Verification items for the finished model (mm, model axes). A direction names the side the tool comes from. Round coordinates to 2 decimals unless told otherwise and drop trailing zeros. Order: outer loops, then holes, each group sorted by start corner. A loop starts at its lowest first (then second) coordinate and runs counter-clockwise, first axis right, second up. Notation, with made-up numbers: M 25.25,16 L 60.25,16 A5 cw 60.25,21 Z; hole C 55,-23 d2. An arc over 180 degrees is marked long. Answer as a JSON object with one key per item and string values. Group by question number.
```python
from build123d import *
from build123d.topology import SkipClean

# Parameters (mm, degrees)
SKETCH_1_R                       = 40
EXTRUDE_1_DEPTH                  = 150
SKETCH_2_R                       = 55
EXTRUDE_2_DEPTH                  = 50
SKETCH_3_R                       = 30
CUT_EXTRUDE_2_DEPTH              = 200
CUT_EXTRUDE_3_DEPTH              = 134
CUT_EXTRUDE_3_DEPTH_BACK         = 106
SKETCH_5_R                       = 6
EXTRUDE_3_DEPTH                  = 45
SKETCH_15_R                      = 50
EXTRUDE_5_DEPTH                  = 20
EXTRUDE_6_DEPTH                  = 59.991870163
SKETCH_17_R                      = 40
EXTRUDE_7_DEPTH                  = 30
SKETCH_18_R                      = 26
CUT_EXTRUDE_25_DEPTH             = 30
SKETCH_19_R                      = 17
CUT_EXTRUDE_26_DEPTH             = 51
CUT_EXTRUDE_27_DEPTH             = 170
CUT_EXTRUDE_27_DEPTH_BACK        = 99
SKETCH_20_R                      = 30
SKETCH_21_R                      = 25
CUT_EXTRUDE_28_DEPTH             = 60
EXTRUDE_8_DEPTH                  = 28
EXTRUDE_8_DEPTH_BACK             = 28
SKETCH_23_R                      = 8.294671539
CUT_EXTRUDE_29_DEPTH             = 70
CUT_EXTRUDE_30_REACH             = 185.367
CUT_EXTRUDE_30_END_RADIUS        = 55
SKETCH_24_W                      = 85
SKETCH_24_H                      = 25
CUT_EXTRUDE_30_DIRECTION_2_DEPTH = 70
CUT_EXTRUDE_31_DEPTH             = 70
CUT_EXTRUDE_31_DEPTH_BACK        = 70
SKETCH_25_W                      = 85
SKETCH_25_H                      = 25
SKETCH_26_R                      = 26
CUT_EXTRUDE_32_DEPTH             = 30
SKETCH_27_R                      = 17
CUT_EXTRUDE_33_DEPTH             = 55
CUT_EXTRUDE_34_DEPTH             = 417
CUT_EXTRUDE_34_DEPTH_BACK        = 195
SKETCH_29_R                      = 30


with BuildPart() as part:
    # 草图1 → 凸台-拉伸1 (new body)
    with BuildSketch(Plane(origin=(0, 0, 0), x_dir=(0, 0, -1), z_dir=(1, 0, 0))):
        Circle(SKETCH_1_R)
    extrude(amount=EXTRUDE_1_DEPTH)

    # 草图2 → 凸台-拉伸2 (add)
    with BuildSketch(Plane(origin=(0, 0, 0), x_dir=(0, 0, -1), z_dir=(1, 0, 0))):
        Circle(SKETCH_2_R)
    extrude(amount=-EXTRUDE_2_DEPTH)

    # 草图3 → 切除-拉伸2 (cut)
    with BuildSketch(Plane(origin=(150, 0, 0), x_dir=(0, 0, -1), z_dir=(1, 0, 0))):
        Circle(SKETCH_3_R)
    extrude(amount=-CUT_EXTRUDE_2_DEPTH, mode=Mode.SUBTRACT)

    # 草图5 → 切除-拉伸3 (cut, two sides: drawn at the far end of the back side and taken through both)
    with BuildSketch(Plane.XY.offset(-CUT_EXTRUDE_3_DEPTH_BACK)):
        with Locations((-25, 0)):
            Circle(SKETCH_5_R)
    extrude(amount=CUT_EXTRUDE_3_DEPTH + CUT_EXTRUDE_3_DEPTH_BACK, mode=Mode.SUBTRACT)

    # 草图7 → 凸台-拉伸3 (add)
    with BuildSketch(Plane(origin=(0, 0, 0), x_dir=(1, 0, 0), z_dir=(0, 1, 0))):
        with BuildLine():
            Line((82.442023832, 21.548591956), (100.118268858, 21.548591956))
            ThreePointArc((100.118268858, 21.548591956), (105, 0), (100.118268858, -21.548591956))
            Line((100.118268858, -21.548591956), (82.442023832, -21.548591956))
            ThreePointArc((82.442023832, -21.548591956), (55, -34.891352615), (27.557976168, -21.548591956))
            Line((27.557976168, -21.548591956), (9.881731142, -21.548591956))
            ThreePointArc((9.881731142, -21.548591956), (5, 0), (9.881731142, 21.548591956))
            Line((9.881731142, 21.548591956), (27.557976168, 21.548591956))
            ThreePointArc((27.557976168, 21.548591956), (55, 34.891352615), (82.442023832, 21.548591956))
        make_face()
    extrude(amount=EXTRUDE_3_DEPTH)

    # 草图15 → 凸台-拉伸5 (add)
    with SkipClean():  # the faces are left unmerged after this step: merging them gives an invalid solid
        with BuildSketch(Plane(origin=(0, 45, 0), x_dir=(1, 0, 0), z_dir=(0, 1, 0))):
            with Locations(Location((55, 0, 0), (0, 0, 154.470748686))):
                Circle(SKETCH_15_R)
        extrude(amount=EXTRUDE_5_DEPTH)

    # 草图16 → 凸台-拉伸6 (add)
    with SkipClean():  # the faces are left unmerged after this step: merging them gives an invalid solid
        with BuildSketch(Plane(origin=(0, 0, 0), x_dir=(1, 0, 0), z_dir=(0, 1, 0))):
            with BuildLine():
                Line((30.539216555, 13.626080627), (17.392421951, 13.626080627))
                ThreePointArc((17.392421951, 13.626080627), (15, 0), (17.392421951, -13.626080627))
                Line((17.392421951, -13.626080627), (30.539216555, -13.626080627))
                ThreePointArc((30.539216555, -13.626080627), (55, -28), (79.460783445, -13.626080627))
                Line((79.460783445, -13.626080627), (92.607578049, -13.626080627))
                ThreePointArc((92.607578049, -13.626080627), (95, 0), (92.607578049, 13.626080627))
                Line((92.607578049, 13.626080627), (79.460783445, 13.626080627))
                ThreePointArc((79.460783445, 13.626080627), (55, 28), (30.539216555, 13.626080627))
            make_face()
        extrude(amount=-EXTRUDE_6_DEPTH)

    # 草图17 → 凸台-拉伸7 (add)
    with BuildSketch(Plane.XZ.offset(59.991870163)):
        with Locations(Location((55, 0, 0), (0, 0, 19.916603358))):
            Circle(SKETCH_17_R)
    extrude(amount=EXTRUDE_7_DEPTH)

    # 草图18 → 切除-拉伸25 (cut)
    with BuildSketch(Plane.XZ.offset(89.991870163)):
        with Locations(Location((55, 0, 0), (0, 0, 270))):
            Circle(SKETCH_18_R)
    extrude(amount=-CUT_EXTRUDE_25_DEPTH, mode=Mode.SUBTRACT)

    # 草图19 → 切除-拉伸26 (cut)
    with BuildSketch(Plane.XZ.offset(59.991870163)):
        with Locations(Location((55, 0, 0), (0, 0, 270))):
            Circle(SKETCH_19_R)
    extrude(amount=-CUT_EXTRUDE_26_DEPTH, mode=Mode.SUBTRACT)

    # 草图20 → 切除-拉伸27 (cut, two sides: drawn at the far end of the back side and taken through both)
    with BuildSketch(Plane(origin=(0, 0, 0), x_dir=(0, 0, -1), z_dir=(1, 0, 0)).offset(-CUT_EXTRUDE_27_DEPTH_BACK)):
        Circle(SKETCH_20_R)
    extrude(amount=CUT_EXTRUDE_27_DEPTH + CUT_EXTRUDE_27_DEPTH_BACK, mode=Mode.SUBTRACT)

    # 草图21 → 切除-拉伸28 (cut)
    with BuildSketch(Plane(origin=(0, 65, 0), x_dir=(1, 0, 0), z_dir=(0, 1, 0))):
        with Locations(Location((55, 0, 0), (0, 0, 270))):
            Circle(SKETCH_21_R)
    extrude(amount=-CUT_EXTRUDE_28_DEPTH, mode=Mode.SUBTRACT)

    # 草图22 → 凸台-拉伸8 (add, two sides: drawn at the far end of the back side and taken through both)
    with BuildSketch(Plane.XY.offset(-EXTRUDE_8_DEPTH_BACK)):
        with BuildLine():
            Line((119.756495452, -72.615787856), (55, -72.615787856))
            Line((55, -72.615787856), (55, -17.615787856))
            Line((55, -17.615787856), (134.756495452, -17.615787856))
            Line((134.756495452, -17.615787856), (134.756495452, -57.615787856))
            ThreePointArc((134.756495452, -57.615787856), (130.36309717, -68.222389574), (119.756495452, -72.615787856))
        make_face()
    extrude(amount=EXTRUDE_8_DEPTH + EXTRUDE_8_DEPTH_BACK)

    # 草图23 → 切除-拉伸29 (cut)
    with BuildSketch(Plane.XY.offset(28)):
        with Locations((118.599166742, -58.702167389)):
            Circle(SKETCH_23_R)
    extrude(amount=-CUT_EXTRUDE_29_DEPTH, mode=Mode.SUBTRACT)

    # 切除-拉伸30: up to this cylinder (the profile starts inside it)
    cut_extrude_30_end = Plane(origin=(-27.5, 0, 0), z_dir=(1, 0, 0)) * Cylinder(CUT_EXTRUDE_30_END_RADIUS, 481.734, mode=Mode.PRIVATE)
    # 草图24 → 切除-拉伸30 (cut, up to the surface)
    with BuildSketch(Plane(origin=(0, 0, 0), x_dir=(1, 0, 0), z_dir=(0, 1, 0)), mode=Mode.PRIVATE) as cut_extrude_30_sk1:
        with Locations((-27.5, -47.5)):
            Rectangle(SKETCH_24_W, SKETCH_24_H)
    cut_extrude_30_tool1 = extrude(cut_extrude_30_sk1.sketch, amount=-CUT_EXTRUDE_30_REACH, mode=Mode.PRIVATE) & cut_extrude_30_end
    add(cut_extrude_30_tool1.solids().sort_by_distance((-27.5, 0, 47.5))[0], mode=Mode.SUBTRACT)

    # 草图24 → 切除-拉伸30 direction 2 (cut)
    with BuildSketch(Plane(origin=(0, 0, 0), x_dir=(1, 0, 0), z_dir=(0, 1, 0))):
        with Locations((-27.5, -47.5)):
            Rectangle(SKETCH_24_W, SKETCH_24_H)
    extrude(amount=CUT_EXTRUDE_30_DIRECTION_2_DEPTH, mode=Mode.SUBTRACT)

    # 草图25 → 切除-拉伸31 (cut, two sides: drawn at the far end of the back side and taken through both)
    with BuildSketch(Plane(origin=(0, 0, 0), x_dir=(1, 0, 0), z_dir=(0, 1, 0)).offset(-CUT_EXTRUDE_31_DEPTH_BACK)):
        with Locations((-27.5, 47.5)):
            Rectangle(SKETCH_25_W, SKETCH_25_H)
    extrude(amount=CUT_EXTRUDE_31_DEPTH + CUT_EXTRUDE_31_DEPTH_BACK, mode=Mode.SUBTRACT)

    # 草图26 → 切除-拉伸32 (cut)
    with BuildSketch(Plane.XZ.offset(89.991870163)):
        with Locations(Location((55, 0, 0), (0, 0, 270))):
            Circle(SKETCH_26_R)
    extrude(amount=-CUT_EXTRUDE_32_DEPTH, mode=Mode.SUBTRACT)

    # 草图27 → 切除-拉伸33 (cut)
    with BuildSketch(Plane.XZ.offset(59.991870163)):
        with Locations(Location((55, 0, 0), (0, 0, 270))):
            Circle(SKETCH_27_R)
    extrude(amount=-CUT_EXTRUDE_33_DEPTH, mode=Mode.SUBTRACT)

    # 草图29 → 切除-拉伸34 (cut, two sides: drawn at the far end of the back side and taken through both)
    with BuildSketch(Plane(origin=(0, 0, 0), x_dir=(0, 0, -1), z_dir=(1, 0, 0)).offset(-CUT_EXTRUDE_34_DEPTH_BACK)):
        Circle(SKETCH_29_R)
    extrude(amount=CUT_EXTRUDE_34_DEPTH + CUT_EXTRUDE_34_DEPTH_BACK, mode=Mode.SUBTRACT)


solid = part.part
```
Q1. Thickness scan on line 1 (Z direction, x = 55, y = -53); line 2 (X direction, y = -61, z = -17); line 3 (X direction, y = 48.5, z = -4.5). Record the ranges inside material, lowest first. Write a range as from..to.
Q2. Cross-section at A-A, the plane x = -25. Record the cut outline in (y, z), then the cut area to 3 significant figures.
Q3. Cross-section at D-D, the plane x = -4. Record the cut outline in (y, z).
Q4. Cross-section at C-C, the plane y = 0. Record the cut outline in (x, z).
Q5. Gauge pin test, flat ends, axial feed: pin 1 Ø4 at (x, y) = (98, -34) entering from -Z; pin 2 Ø6 at (x, y) = (-29, -50) entering from -Z; pin 3 Ø12 at (x, y) = (-23, -20) entering from -Z; pin 4 Ø9.5 at (x, y) = (-25, 0) entering from +Z. Record the tip position at first contact, or that the pin passes through.
Q6. Release check for a two-part mould opening along X. For faces 1 (the face through (52, 45, -35)), 2 (the face through (134.756, -46, 0)), 3 (the face through (47, -59.992, -30)) record: released by +X, released by -X, zero draft, split by the parting line, or undercut.
Q7. Cross-section at B-B, the plane z = -32.5. Record the cut outline in (x, y), then the cut area to 3 significant figures.
Q8. Tool access check on faces 4 (the face through (-18, -1, -35)), 5 (the face through (55.44, 34.93, 34.89)), 6 (the face through (15, 0, 37)), 7 (the face through (45.42, 46.51, 23.09)). Record the directions out of +Z, -Z, +X, -X, +Y, -Y that give a thin tool (end or side, any length) a straight path to the whole face; none if there is none.
Conclusion:
{
 "1": {"line 1": "-28..-17, 17..28", "line 2": "18.79..35.33, 74.67..110.63, 126.57..134.37", "line 3": "-50..0, 5.2..30.41, 79.59..104.8"},
 "2": {"outline": "M -42.43,-35 L -6,-35 L -6,-29.39 A30 cw -6,29.39 L -6,35 L -42.43,35 A55 ccw Z; M 6,-35 L 42.43,-35 A55 ccw 42.43,35 L 6,35 L 6,29.39 A30 cw 6,-29.39 Z", "area": "4,190 mm2"},
 "3": {"outline": "M -42.43,-35 L 42.43,-35 A55 ccw 42.43,35 L -42.43,35 A55 ccw Z; hole C 0,0 d60"},
 "4": {"outline": "M -50,-35 L -31,-35 L -31,-30 L -50,-30 Z; M -50,30 L -31,30 L -31,35 L -50,35 Z; M -19,-35 L 15,-35 L 15,-40 L 150,-40 L 150,-30 L -19,-30 Z; M -19,30 L 150,30 L 150,40 L 15,40 L 15,35 L -19,35 Z"},
 "5": {"pin 1": "z = -28", "pin 2": "z = -28.57", "pin 3": "z = -35", "pin 4": "through"},
 "6": {"face 1": "undercut", "face 2": "released by +X", "face 3": "zero draft"},
 "7": {"outline": "M -50,-44.37 L 0,-44.37 L 0,-23.32 L 150,-23.32 L 150,23.32 L 67.69,23.32 L 67.69,45 L 93,45 L 93,65 L 17,65 L 17,45 L 42.31,45 L 42.31,23.32 L 0,23.32 L 0,44.37 L -50,44.37 Z; M 31.68,-89.99 L 78.32,-89.99 L 78.32,-59.99 L 31.68,-59.99 Z; hole C -25,0 d12", "area": "14,800 mm2"},
 "8": {"face 4": "-Z, -X, +Y, -Y", "face 5": "+Z", "face 6": "+Z, -X, +Y, -Y", "face 7": "+Y"}
}
